Check sheet for the modelled part. Datum: model origin and axes. Units: mm. A direction names the side the tool comes from. Round coordinates to 2 decimals unless told otherwise and drop trailing zeros. Loops run counter-clockwise (first coordinate to the right, second up) from the corner with the lowest first, then second, coordinate; pieces in that order, holes last. Notation, with made-up numbers: (44.5, -34) - (75.5, -34) arc R24 ccw to (75.5, -17) - close; hole circle Ø10 at (27.25, -20). An arc over 180 degrees is marked (long way). Return JSON: item names as keys, results as strings.
from build123d import *

# Parameters (mm, degrees)
SKETCH2_R           = 1.4224
BOSS_EXTRUDE1_DEPTH = 15.875
CUT_EXTRUDE1_DEPTH  = 43.817135594


with BuildPart() as part:
    # Sketch1 → Base-Revolve (revolve)
    with BuildSketch(Plane(origin=(0, 0, 0), x_dir=(0, 0, -1), z_dir=(1, 0, 0))):
        with BuildLine():
            Line((-22.86, 15.282157927), (-20.7264, 15.282157927))
            ThreePointArc((-20.7264, 15.282157927), (-21.322188128, 17.024235032), (-22.86, 18.036623683))
            Line((-22.86, 18.036623683), (-22.86, 15.282157927))
        make_face()
    revolve(axis=Axis((0, 15.282157927, 28.59405), (0, 0, -1)))

    # Sketch2 → Boss-Extrude1 (add)
    with BuildSketch(Plane.XY.offset(22.86)):
        with Locations(Location((0, 15.24, 0), (0, 0, 180))):
            Circle(SKETCH2_R)
    extrude(amount=BOSS_EXTRUDE1_DEPTH)

    # Sketch4 → Cut-Extrude1 (cut, through all)
    with BuildSketch(Plane(origin=(0, 0, 0), x_dir=(0, 0, -1), z_dir=(1, 0, 0))):
        with BuildLine():
            Line((-22.171112501, 14.926557927), (-20.748712501, 14.926557927))
            ThreePointArc((-20.748712501, 14.926557927), (-20.7264, 15.282157927), (-20.748712501, 15.637757927))
            Line((-20.748712501, 15.637757927), (-22.171112501, 15.637757927))
            Line((-22.171112501, 15.637757927), (-22.171112501, 14.926557927))
        make_face()
    cut_extrude1 = extrude(amount=-CUT_EXTRUDE1_DEPTH, mode=Mode.SUBTRACT)

    # Mirror1: Cut-Extrude1 across plane
    add(cut_extrude1.mirror(Plane(origin=(0, 15.282157927, 23.5712), x_dir=(0, 0, 1), z_dir=(1, 0, 0))), mode=Mode.SUBTRACT)


solid = part.part
Q1. Tool access check on faces 1 (the face through (0, 15, 38.735)), 2 (the face through (0, 14.927, 22)). Record the directions out of +Z, -Z, +X, -X, +Y, -Y that give a thin tool (end or side, any length) a straight path to the whole face; none if there is none.
Answer key:
{"face 1": "+Z, +X, -X, +Y, -Y", "face 2": "-Z, +X, -X"}
Q2. Sectioned sample at A-A (x = 0). Enter the section's corners in (y, z) (3 decimals), plus the area to 3 significant figures.
Answer key:
{"outline": "(12.528, 22.86) arc R2.845 ccw to (14.927, 20.749) - (14.927, 22.171) - (15.638, 22.171) - (15.638, 20.749) arc R2.845 ccw to (18.037, 22.86) - (16.662, 22.86) - (16.662, 38.735) - (13.818, 38.735) - (13.818, 22.86) - close", "area": "52.8 mm²"}
Q3. Depth check by flat-ended pin: P1, Ø3, axis at y = 15, z = 34, coming from the -X side; P2, Ø0.6, axis at x = 0.5, y = 15, coming from the -Z side; P3, Ø1.1, axis at x = 0.5, z = 21, coming from the -Y side. Enter the tip coordinate at first touch or a pass-through.
Answer key:
{"P1": "stops at x = -1.42", "P2": "stops at z = 20.76", "P3": "stops at y = 13.33"}
Q4. Draft check along Y on faces 3 (the face through (0, 15.638, 22)), 4 (the face through (-1.2, 16.5, 22.86)), 5 (the face through (0.31, 16.63, 30.69)). Enter one of: released by +Y, released by -Y, zero draft, split by the parting line, or undercut.
Answer key:
{"face 3": "undercut", "face 4": "zero draft", "face 5": "split by the parting line"}
Q5. Sectioned sample at D-D (x = 1.1). Enter the section's corners in (y, z) (3 decimals).
Answer key:
{"outline": "(12.757, 22.86) arc R2.624 ccw to (14.927, 20.972) - (14.927, 22.171) - (15.638, 22.171) - (15.638, 20.972) arc R2.624 ccw to (17.807, 22.86) - (16.142, 22.86) - (16.142, 38.735) - (14.338, 38.735) - (14.338, 22.86) - close"}
Q6. Sectioned sample at B-B (y = 15.24). Enter the section's corners in (x, z) (3 decimals), plus the area to 3 significant figures.
Answer key:
{"outline": "(-2.754, 22.86) arc R2.844 ccw to (-2.476, 22.171) - (2.476, 22.171) arc R2.844 ccw to (2.754, 22.86) - (1.422, 22.86) - (1.422, 38.735) - (-1.422, 38.735) - (-1.422, 22.86) - close", "area": "48.8 mm²"}
Q7. Sectioned sample at C-C (z = 27). Enter the section's corners in (x, y).
Answer key:
{"outline": "circle Ø2.84 at (0, 15.24)"}
Q8. Scan lines: probe 1 along Z at (x, y) = (0.15, 15.2) (3 decimals); probe 2 along Z at (x, y) = (-2.2, 15.3); probe 3 along X at (y, z) = (15.25, 31). Record each from-to range of solid material in increasing order. Write a range as [from, to].
Answer key:
{"probe 1": "z = [22.171, 38.735]", "probe 2": "z = [22.17, 22.86]", "probe 3": "x = [-1.42, 1.42]"}
